For this review, use the dimensioned drawing (mm, ordinates from the lowest corner) and the shaded views. Coordinates: 2 decimals unless noted, no trailing zeros. Loops run counter-clockwise (first coordinate to the right, second up) from the corner with the lowest first, then second, coordinate; pieces in that order, holes last. Notation, with made-up numbers: (-4, 7) -> (11, 7) arc R27 cw to (11, 42) -> close; hole circle Ø4 at (32.5, -14.5). An arc over 180 degrees is marked (long way). Use one line per item in the form item = value. Start each with the question number.
1. For pin 1 (1.5 mm diameter, centred on y = 12, z = 6, fed in from -X); pin 2 (2 mm diameter, centred on x = 38.5, z = 17, fed in from +Y), all flat-tipped, find the tip position at first contact; note any pin that passes through.
2. Wall thickness on line 1 (Y direction, x = 22.5, z = 20.5); line 2 (Y direction, x = 52, z = 5); line 3 (X direction, y = 37, z = 21.75) (1 decimal): over which ranges is each line inside the solid? List them lowest first. Write a range as from..to.
3. Consider section A-A (z = 14.5). State the section outline as (x, y) points.
4. The part is to be moulded in two halves that separate along Y. For the marked faces 1, 2 and 3, say which applies: released by +Y, released by -Y, zero draft, split by the parting line, or undercut.
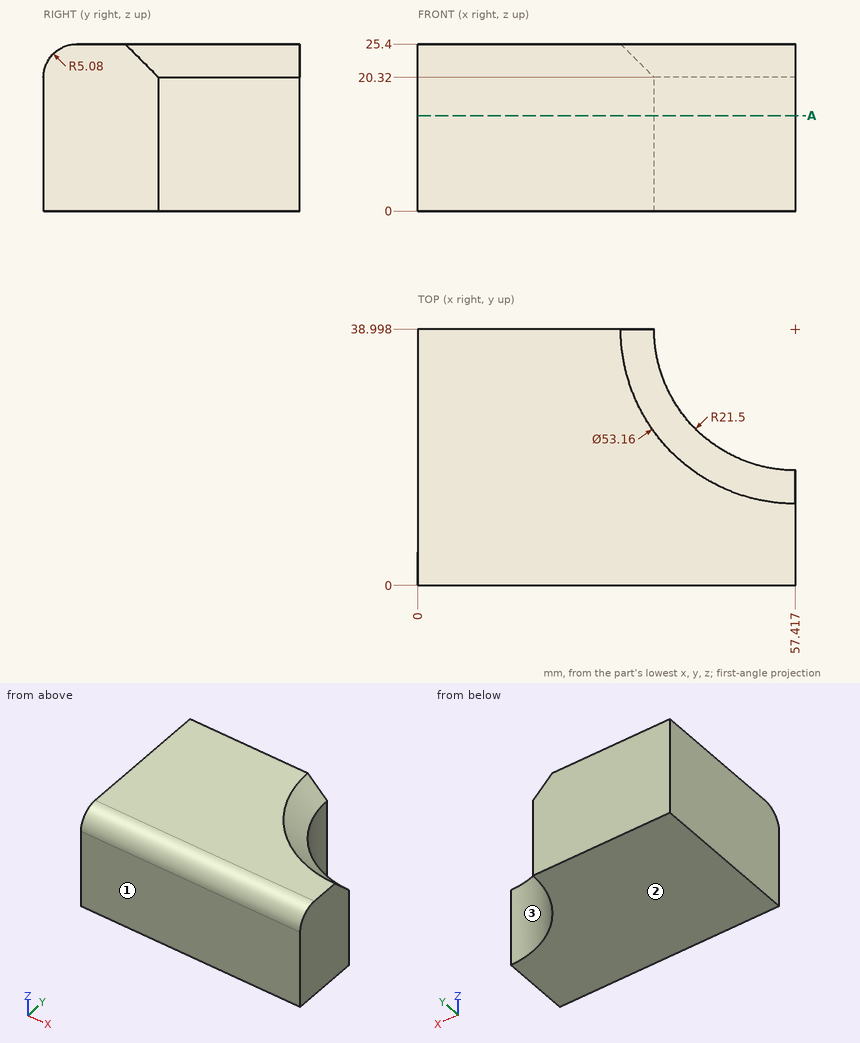
Geometry check:
q1.pin_1 = 0
q1.pin_2 = 30.9
q2.line_1 = 0..39
q2.line_2 = 0..18.19
q2.line_3 = 0..34.6
q3.outline = (0, 0) -> (57.42, 0) -> (57.42, 17.5) arc R21.5 cw to (35.92, 39) -> (0, 39) -> close
q4.face_1 = released by -Y
q4.face_2 = zero draft
q4.face_3 = released by +Y
